Source: CAD feature listing. Evaluate the final solid. Frame: model axes, mm. A direction names the side the tool comes from. Round coordinates to 2 decimals unless told otherwise and drop trailing zeros. Order: outer loops, then holes, each group sorted by start corner. A loop starts at its lowest first (then second) coordinate and runs counter-clockwise, first axis right, second up. Notation, with made-up numbers: (13.25, 87.25) - (22.25, 87.25) arc R19 cw to (22.25, 106.25) - close; hole circle Ø11 at (25.5, 12). An arc over 180 degrees is marked (long way). Return JSON: item names as keys, results as strings. Group by question number.
1) Ray query, line 1 (X direction, y = 236, z = 168.5); line 2 (X direction, y = 275.5, z = 124); line 3 (Z direction, x = 236, y = 70.5). Return the intervals inside material, ascending. Write a range as from..to.
2) Access query for faces 4 (the flat face through (248, 241.3, 13)), 5 (the flat face through (-228.6, 182, 88)), 6 (the flat face through (260, 135, 152.4)). Directions: +Z, -Z, +X, -X, +Y, -Y. A direction counts if a zero-diameter tool reaches every point of the face in a straight line with its end or side. Return the directions, or none.
3) Section D-D, the plane y = 166. Return loops of the section in (x, z), plus the area to 3 significant figures.
4) Section C-C, the plane z = 164.5. Return loops of the section in (x, y) (3 decimals), plus the area to 3 significant figures.
5) Section A-A, the plane y = 98.5. Return loops of the section in (x, z), plus the area to 3 significant figures.
6) Section B-B, the plane y = 267. Return loops of the section in (x, z).
7) Contact query for a flat-ended pin moving along its axis: P1, Ø11.5, axis at x = -31.87, y = 34.8, coming from the +Z side (3 decimals). Output: stop coordinate, or through.
8) Mould query, pull axis Z, two halves, no side actions, for faces 1 (the flat face through (248, 241.3, 165)), 2 (the flat face through (-4, 52, 0)), 3 (the flat face through (34, 69.597, 88)). Classes: pulls with the +Z half, pulls with the -Z half, needs draft (parallel to the pull), parting line crosses it, or undercut.
```python
from build123d import *

# Parameters (mm, degrees)
BOSS_EXTRUDE1_DEPTH = 177.8
SKETCH4_R           = 25.4
SKETCH4_R_2         = 15.875
SKETCH4_R_3         = 6.35
CUT_EXTRUDE1_DEPTH  = 462.992536298
SKETCH5_W           = 127
SKETCH5_H           = 171.70338098
CUT_EXTRUDE2_DEPTH  = 605.86044142


with BuildPart() as part:
    # Sketch1 → Boss-Extrude1 (new body)
    with BuildSketch(Plane.XY):
        Polygon((-304.8, 0), (304.8, 0), (304.8, 241.3), (190.5, 241.3), (190.5, 69.59661902), (-228.6, 69.59661902), (-228.6, 298.19661902), (-304.8, 298.19661902), align=None)
    extrude(amount=BOSS_EXTRUDE1_DEPTH)

    # Sketch4 → Cut-Extrude1 (cut, through all)
    with BuildSketch(Plane.XY.offset(177.8)):
        with Locations((244.103977456, 159.533856411)):
            Circle(SKETCH4_R)
        with Locations((-268.663213375, 276.196433082)):
            Circle(SKETCH4_R_2)
        with Locations((-31.867387375, 34.79830951)):
            Circle(SKETCH4_R_3)
    extrude(amount=-CUT_EXTRUDE1_DEPTH, mode=Mode.SUBTRACT)

    # Sketch5 → Cut-Extrude2 (cut, through all)
    with BuildSketch(Plane.ZY.offset(-190.5)):
        with Locations((88.9, 155.44830951)):
            Rectangle(SKETCH5_W, SKETCH5_H)
    extrude(amount=-CUT_EXTRUDE2_DEPTH, mode=Mode.SUBTRACT)


solid = part.part
```
Geometry check:
{
 "1": {"line 1": "-304.8..-228.6, 190.5..304.8", "line 2": "-304.8..-284.52, -252.8..-228.6", "line 3": "0..25.4, 152.4..177.8"},
 "2": {"face 4": "+Z, -Z, +X, +Y", "face 5": "+Z, -Z, +Y", "face 6": "+X, +Y"},
 "3": {"outline": "(-304.8, 0) - (-228.6, 0) - (-228.6, 177.8) - (-304.8, 177.8) - close; (190.5, 0) - (219.54, 0) - (219.54, 25.4) - (190.5, 25.4) - close; (190.5, 152.4) - (219.54, 152.4) - (219.54, 177.8) - (190.5, 177.8) - close; (268.67, 0) - (304.8, 0) - (304.8, 25.4) - (268.67, 25.4) - close; (268.67, 152.4) - (304.8, 152.4) - (304.8, 177.8) - (268.67, 177.8) - close", "area": "16,900 mm2"},
 "4": {"outline": "(-304.8, 0) - (304.8, 0) - (304.8, 241.3) - (190.5, 241.3) - (190.5, 69.597) - (-228.6, 69.597) - (-228.6, 298.197) - (-304.8, 298.197) - close; hole circle Ø31.75 at (-268.663, 276.196); hole circle Ø12.7 at (-31.867, 34.798); hole circle Ø50.8 at (244.104, 159.534)", "area": "76,500 mm2"},
 "5": {"outline": "(-304.8, 0) - (-228.6, 0) - (-228.6, 177.8) - (-304.8, 177.8) - close; (190.5, 0) - (304.8, 0) - (304.8, 25.4) - (190.5, 25.4) - close; (190.5, 152.4) - (304.8, 152.4) - (304.8, 177.8) - (190.5, 177.8) - close", "area": "19,400 mm2"},
 "6": {"outline": "(-304.8, 0) - (-281.6, 0) - (-281.6, 177.8) - (-304.8, 177.8) - close; (-255.72, 0) - (-228.6, 0) - (-228.6, 177.8) - (-255.72, 177.8) - close"},
 "7": {"P1": "through"},
 "8": {"face 1": "needs draft", "face 2": "pulls with the -Z half", "face 3": "undercut"}
}
